Study the drawing (mm; zero at the part's minimum x, y, z) and answer. Coordinates: 2 decimals unless noted, no trailing zeros. Order: outer loops, then holes, each group sorted by start corner. A loop starts at its lowest first (then second) coordinate and runs counter-clockwise, first axis right, second up. Notation, with made-up numbers: (17, 51) -> (26, 51) arc R20 ccw to (26, 73) -> close; hole circle Ø5 at (73.25, 36). An arc over 180 degrees is marked (long way). Write each question's results on one line, items separated by ' | '. Start each with the question number.
(1) Given pin 1 (1.6 mm diameter, centred on x = 2, y = 47.5, fed in from -Z); pin 2 (1.6 mm diameter, centred on x = 1.5, z = 16.5, fed in from -Y); pin 3 (23 mm diameter, centred on y = 127, z = 76.2, fed in from +X), each flat-ended and moving along its own axis, determine where each tip first touches the part or whether it passes through.
(2) Straight lines are drawn through the part: L1, parallel to Z at x = 0.1, y = 23; L2, parallel to Y at x = 1.35, z = 139.7; L3, parallel to Y at x = 1.9, z = 135. For each, find the intervals that lie inside material, in ascending order.
(3) The part is cut by section D-D, the plane y = 16.5. Give the vertices of the cut face in (x, z) (3 decimals).
(4) The part is cut by section B-B, the plane z = 61. Give the vertices of the cut face in (x, y) (3 decimals), then the cut area to 3 significant figures.
(5) The part is cut by section C-C, the plane x = 2.3. Give the vertices of the cut face in (y, z).
(6) The part is cut by section A-A, the plane y = 127. Give the vertices of the cut face in (x, z) (3 decimals).
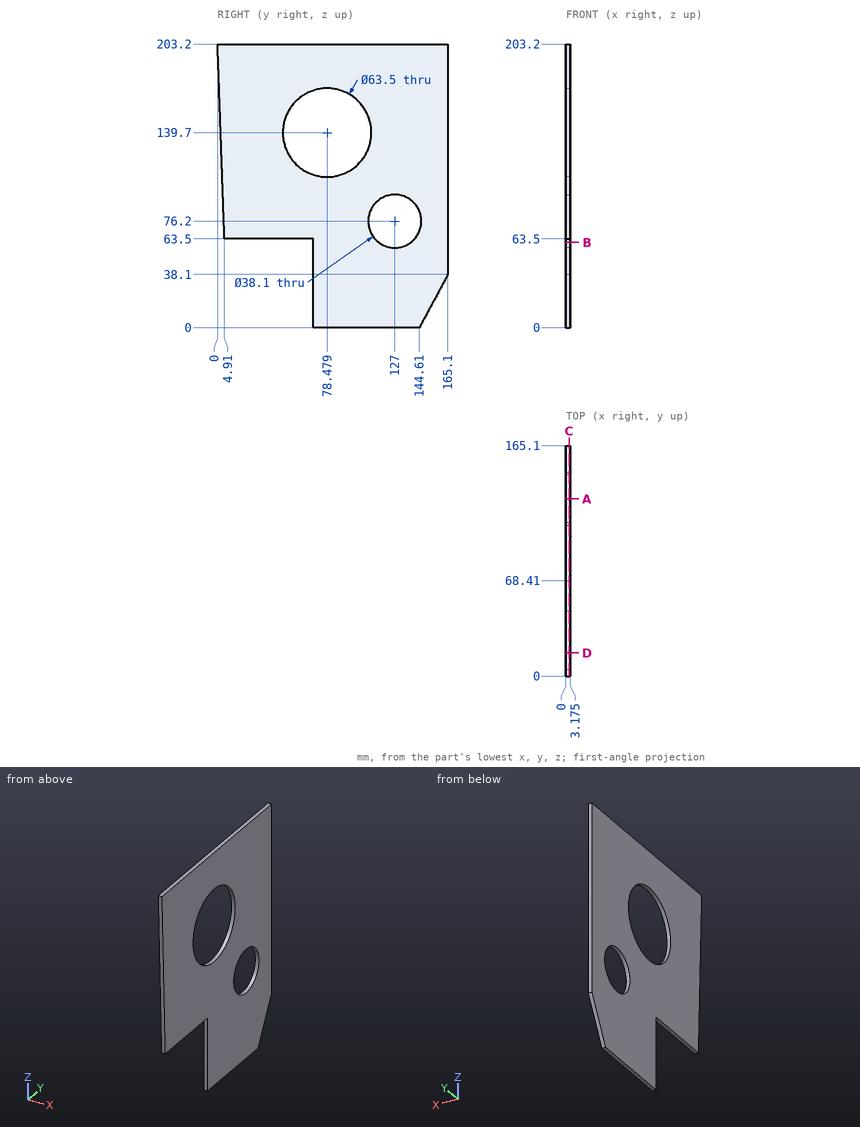
Established:
1) pin 1: stops at z = 63.5 | pin 2: stops at y = 68.41 | pin 3: passes through
2) L1: z = 63.5 to 203.2 | L2: y = 2.23 to 46.73, 110.23 to 165.1 | L3: y = 2.4 to 47.08, 109.88 to 165.1
3) outline: (0, 63.5) -> (3.175, 63.5) -> (3.175, 203.2) -> (0, 203.2) -> close
4) outline: (0, 68.41) -> (3.175, 68.41) -> (3.175, 115.517) -> (0, 115.517) -> close; (0, 138.483) -> (3.175, 138.483) -> (3.175, 165.1) -> (0, 165.1) -> close | area: 234 mm^2
5) outline: (0, 203.2) -> (4.91, 63.5) -> (68.41, 63.5) -> (68.41, 0) -> (144.61, 0) -> (165.1, 38.1) -> (165.1, 203.2) -> close; hole circle Ø63.5 at (78.48, 139.7); hole circle Ø38.1 at (127, 76.2)
6) outline: (0, 0) -> (3.175, 0) -> (3.175, 57.15) -> (0, 57.15) -> close; (0, 95.25) -> (3.175, 95.25) -> (3.175, 203.2) -> (0, 203.2) -> close
